Read the model definition and answer for the solid it produces. Units are mm, in the model's axes. A direction names the side the tool comes from. Coordinates: 2 decimals unless noted, no trailing zeros. Loops run counter-clockwise (first coordinate to the right, second up) from the corner with the lowest first, then second, coordinate; pieces in that order, holes last. Notation, with made-up numbers: (73.25, -0.75) -> (93.25, -0.75) arc R9 ccw to (93.25, 12.25) -> close; hole circle Ø7 at (56, -5.75). An arc over 180 degrees is marked (long way). Answer as a JSON object with one key per item and string values. Group by question number.
1) Section C-C, the plane z = -80 is taken. Give the vertices of the cut face in (x, y).
2) Determine the mould class of faces 4 (the face through (-42.44, 5.07, -24.54)), 5 (the face through (-44, 5, -34)), 6 (the face through (-46.889, 4.93, -93.325)) for opening direction X: released by +X, released by -X, zero draft, split by the parting line, or undercut.
3) Consider probe 1 along Z at (x, y) = (-11.5, 3.75); probe 2 along X at (y, z) = (2, -51.5); probe 3 along X at (y, z) = (5, -24). Determine where each line is inside the solid, lowest interval first. Write a range as [from, to].
4) Which of the six approach directions +Z, -Z, +X, -X, +Y, -Y give full straight-line access (tool end or side, diameter ignored) to faces 1 (the face through (-4, 5, 4)), 2 (the face through (-38.5, 12.46, -75.23)), 3 (the face through (26.677, 4.93, -9.9))?
5) Section A-A, the plane z = 0 is taken. Give the vertices of the cut face in (x, y), plus the area to 3 significant figures.
6) Flat-ended cylindrical pins translate along their axes: P1, Ø1, axis at x = 26.5, y = 4.5, coming from the -Z side; P2, Ø3, axis at y = 5.5, z = -32, coming from the -X side; P3, Ø1, axis at y = 2.5, z = -30, coming from the +X side; P4, Ø8, axis at x = -16, z = 0, coming from the -Y side. Find the tip coordinate at first contact, or state that the pin passes through.
7) Section D-D, the plane y = 11.5 is taken. Give the vertices of the cut face in (x, z), plus the area to 3 significant figures.
8) Section B-B, the plane x = -40 is taken. Give the vertices of the cut face in (y, z), plus the area to 3 significant figures.
from build123d import *

# Parameters (mm, degrees)
BOSS_EXTRUDE1_DEPTH = 10
SKETCH2_R           = 5
BOSS_EXTRUDE2_DEPTH = 5
SKETCH3_R           = 5
BOSS_EXTRUDE3_DEPTH = 5
SKETCH4_R           = 2.5
CUT_EXTRUDE1_DEPTH  = 111.227038425
SKETCH5_R           = 2.5
CUT_EXTRUDE2_DEPTH  = 111.227038425
SKETCH6_R           = 2.5
CUT_EXTRUDE3_DEPTH  = 111.227038425
SKETCH7_R           = 2.5
CUT_EXTRUDE4_DEPTH  = 111.227038425
SKETCH8_R           = 2.5
CUT_EXTRUDE5_DEPTH  = 111.227038425
CUT_EXTRUDE6_DEPTH  = 111.227038425
FILLET3_R           = 3
SKETCH11_R          = 2.5
CUT_EXTRUDE7_DEPTH  = 111.227038425
SKETCH12_R          = 2.5
CUT_EXTRUDE8_DEPTH  = 111.227038425
FILLET4_R           = 3
FILLET5_R           = 3
FILLET6_R           = 3
FILLET7_R           = 3
FILLET8_R           = 10


with BuildPart() as part:
    # Sketch1 → Boss-Extrude1 (new body)
    with BuildSketch(Plane(origin=(0, 0, 0), x_dir=(1, 0, 0), z_dir=(0, 1, 0))):
        with BuildLine():
            Line((-25.590058181, 75.834237552), (36, 14.456832295))
            ThreePointArc((36, 14.456832295), (53.050951275, -7.394097025), (25.543167705, -4))
            Line((25.543167705, -4), (-44, -4))
            Line((-44, -4), (-44, 65.543167705))
            ThreePointArc((-44, 65.543167705), (-47.31903353, 93.093194728), (-25.590058181, 75.834237552))
        make_face()
    extrude(amount=BOSS_EXTRUDE1_DEPTH)

    # Sketch2 → Boss-Extrude2 (add)
    with BuildSketch(Plane(origin=(0, 10, 0), x_dir=(1, 0, 0), z_dir=(0, 1, 0))):
        with Locations(Location((-40, 80, 0), (0, 0, 270))):
            Circle(SKETCH2_R)
    extrude(amount=BOSS_EXTRUDE2_DEPTH)

    # Sketch3 → Boss-Extrude3 (add)
    with BuildSketch(Plane(origin=(0, 10, 0), x_dir=(1, 0, 0), z_dir=(0, 1, 0))):
        with Locations(Location((40, 0, 0), (0, 0, 270))):
            Circle(SKETCH3_R)
    extrude(amount=BOSS_EXTRUDE3_DEPTH)

    # Sketch4 → Cut-Extrude1 (cut, through all)
    with BuildSketch(Plane(origin=(0, 10, 0), x_dir=(1, 0, 0), z_dir=(0, 1, 0))):
        with Locations(Location((-40, 50, 0), (0, 0, 270))):
            Circle(SKETCH4_R)
    extrude(amount=-CUT_EXTRUDE1_DEPTH, mode=Mode.SUBTRACT)

    # Sketch5 → Cut-Extrude2 (cut, through all)
    with BuildSketch(Plane(origin=(0, 10, 0), x_dir=(1, 0, 0), z_dir=(0, 1, 0))):
        with Locations(Location((-40, 24, 0), (0, 0, 270))):
            Circle(SKETCH5_R)
    extrude(amount=-CUT_EXTRUDE2_DEPTH, mode=Mode.SUBTRACT)

    # Sketch6 → Cut-Extrude3 (cut, through all)
    with BuildSketch(Plane(origin=(0, 10, 0), x_dir=(1, 0, 0), z_dir=(0, 1, 0))):
        with Locations(Location((10, 0, 0), (0, 0, 270))):
            Circle(SKETCH6_R)
    extrude(amount=-CUT_EXTRUDE3_DEPTH, mode=Mode.SUBTRACT)

    # Sketch7 → Cut-Extrude4 (cut, through all)
    with BuildSketch(Plane(origin=(0, 10, 0), x_dir=(1, 0, 0), z_dir=(0, 1, 0))):
        with Locations(Location((-16, 0, 0), (0, 0, 270))):
            Circle(SKETCH7_R)
    extrude(amount=-CUT_EXTRUDE4_DEPTH, mode=Mode.SUBTRACT)

    # Sketch8 → Cut-Extrude5 (cut, through all)
    with BuildSketch(Plane(origin=(0, 10, 0), x_dir=(1, 0, 0), z_dir=(0, 1, 0))):
        with Locations(Location((-36, 4, 0), (0, 0, 270))):
            Circle(SKETCH8_R)
    extrude(amount=-CUT_EXTRUDE5_DEPTH, mode=Mode.SUBTRACT)

    # Sketch10 → Cut-Extrude6 (cut, through all)
    with BuildSketch(Plane(origin=(0, 10, 0), x_dir=(1, 0, 0), z_dir=(0, 1, 0))):
        with BuildLine():
            Line((-36, 74.914042926), (31.145878515, 8))
            Line((31.145878515, 8), (-21.543167705, 8))
            ThreePointArc((-21.543167705, 8), (-26.917048938, 15.937336386), (-36, 19))
            Line((-36, 19), (-36, 74.914042926))
        make_face()
    extrude(amount=-CUT_EXTRUDE6_DEPTH, mode=Mode.SUBTRACT)

    # Fillet3
    fillet3_edges = [part.edges().sort_by_distance(p)[0] for p in [
        (-44, 5, -65.543167705),
    ]]
    fillet(fillet3_edges, radius=FILLET3_R)

    # Sketch11 → Cut-Extrude7 (cut, through all)
    with BuildSketch(Plane(origin=(0, 10, 0), x_dir=(1, 0, 0), z_dir=(0, 1, 0))):
        with Locations(Location((-9.398144918, 54.051141856, 0), (0, 0, 270))):
            Circle(SKETCH11_R)
    extrude(amount=-CUT_EXTRUDE7_DEPTH, mode=Mode.SUBTRACT)

    # Sketch12 → Cut-Extrude8 (cut, through all)
    with BuildSketch(Plane(origin=(0, 10, 0), x_dir=(1, 0, 0), z_dir=(0, 1, 0))):
        with Locations(Location((18.886126329, 25.766870608, 0), (0, 0, 270))):
            Circle(SKETCH12_R)
    extrude(amount=-CUT_EXTRUDE8_DEPTH, mode=Mode.SUBTRACT)

    # Fillet4
    fillet4_edges = [part.edges().sort_by_distance(p)[0] for p in [
        (-36, 5, -74.914042926),
    ]]
    fillet(fillet4_edges, radius=FILLET4_R)

    # Fillet5
    fillet5_edges = [part.edges().sort_by_distance(p)[0] for p in [
        (31.145878515, 5, -8),
    ]]
    fillet(fillet5_edges, radius=FILLET5_R)

    # Fillet6
    fillet6_edges = [part.edges().sort_by_distance(p)[0] for p in [
        (-36, 5, -19),
    ]]
    fillet(fillet6_edges, radius=FILLET6_R)

    # Fillet7
    fillet7_edges = [part.edges().sort_by_distance(p)[0] for p in [
        (-21.543167705, 5, -8),
    ]]
    fillet(fillet7_edges, radius=FILLET7_R)

    # Fillet8
    fillet8_edges = [part.edges().sort_by_distance(p)[0] for p in [
        (-44, 5, 4),
    ]]
    fillet(fillet8_edges, radius=FILLET8_R)


solid = part.part
Determined:
{
 "1": {"outline": "(-55, 0) -> (-25, 0) -> (-25, 10) -> (-35, 10) -> (-35, 15) -> (-45, 15) -> (-45, 10) -> (-55, 10) -> close"},
 "2": {"face 4": "undercut", "face 5": "released by -X", "face 6": "split by the parting line"},
 "3": {"probe 1": "[-61.79, -55.4], [-52.7, -50.5], [-8, 4]", "probe 2": "[-44, -42], [-38, -36], [-12.5, -1.17]", "probe 3": "[-44, -42.5], [-37.5, -36], [15.09, 17.12], [20.65, 26.42]"},
 "4": {"face 1": "+Z, -X, +Y, -Y", "face 2": "+Y", "face 3": "+Y, -Y"},
 "5": {"outline": "(-42, 0) -> (-18.5, 0) -> (-18.5, 10) -> (-42, 10) -> close; (-13.5, 0) -> (7.5, 0) -> (7.5, 10) -> (-13.5, 10) -> close; (12.5, 0) -> (55, 0) -> (55, 10) -> (45, 10) -> (45, 15) -> (35, 15) -> (35, 10) -> (12.5, 10) -> close", "area": "920 mm²"},
 "6": {"P1": "z = -24.42", "P2": "x = -44", "P3": "x = 20.9", "P4": "y = 0"},
 "7": {"outline": "circle Ø10 at (-40, -80); circle Ø10 at (40, 0)", "area": "157 mm²"},
 "8": {"outline": "(0, -95) -> (10, -95) -> (10, -85) -> (15, -85) -> (15, -75) -> (10, -75) -> (10, -52.5) -> (0, -52.5) -> close; (0, -47.5) -> (10, -47.5) -> (10, -26.5) -> (0, -26.5) -> close; (0, -21.5) -> (10, -21.5) -> (10, 2) -> (0, 2) -> close", "area": "920 mm²"}
}
